```python
from build123d import *
from build123d.topology import SkipClean

# Parameters (mm, degrees)
SKETCH1_R           = 4.3
SKETCH1_R_2         = 3.5
BOSS_EXTRUDE1_DEPTH = 0.5
BOSS_EXTRUDE2_DEPTH = 2.5
SKETCH5_R           = 0.5
CUT_EXTRUDE2_DEPTH  = 3
CIRPATTERN1_COUNT   = 4


with BuildPart() as part:
    # Sketch1 → Boss-Extrude1 (new body)
    with BuildSketch(Plane.XY):
        Circle(SKETCH1_R)
        Circle(SKETCH1_R_2, mode=Mode.SUBTRACT)
    extrude(amount=BOSS_EXTRUDE1_DEPTH)

    # Sketch2 → Boss-Extrude2 (add)
    with SkipClean():  # the faces are left unmerged after this step: merging them gives an invalid solid
        with BuildSketch(Plane.XY.offset(0.5)):
            with BuildLine():
                Line((4.010922587, 1.55), (3.138072657, 1.55))
                ThreePointArc((3.138072657, 1.55), (2.474873734, 2.474873734), (1.55, 3.138072657))
                Line((1.55, 3.138072657), (1.55, 4.010922587))
                ThreePointArc((1.55, 4.010922587), (3.040559159, 3.040559159), (4.010922587, 1.55))
            make_face()
            with BuildLine():
                Line((-4.010922587, 1.55), (-3.138072657, 1.55))
                ThreePointArc((-3.138072657, 1.55), (-2.474873734, 2.474873734), (-1.55, 3.138072657))
                Line((-1.55, 3.138072657), (-1.55, 4.010922587))
                ThreePointArc((-1.55, 4.010922587), (-3.040559159, 3.040559159), (-4.010922587, 1.55))
            make_face()
            with BuildLine():
                Line((1.55, -4.010922587), (1.55, -3.138072657))
                ThreePointArc((1.55, -3.138072657), (2.474873734, -2.474873734), (3.138072657, -1.55))
                Line((3.138072657, -1.55), (4.010922587, -1.55))
                ThreePointArc((4.010922587, -1.55), (3.040559159, -3.040559159), (1.55, -4.010922587))
            make_face()
            with BuildLine():
                Line((-4.010922587, -1.55), (-3.138072657, -1.55))
                ThreePointArc((-3.138072657, -1.55), (-2.474873734, -2.474873734), (-1.55, -3.138072657))
                Line((-1.55, -3.138072657), (-1.55, -4.010922587))
                ThreePointArc((-1.55, -4.010922587), (-3.040559159, -3.040559159), (-4.010922587, -1.55))
            make_face()
        extrude(amount=BOSS_EXTRUDE2_DEPTH)

    # Sketch5 → Cut-Extrude2 (cut)
    with SkipClean():  # the faces are left unmerged after this step: merging them gives an invalid solid
        with BuildSketch(Plane(origin=(3.040559159, 3.040559159, 0), x_dir=(0, 0, -1), z_dir=(0.7071067811865499, 0.7071067811865452, 0))):
            with Locations(Location((-2.2, 0, 0), (0, 0, 90))):
                Circle(SKETCH5_R)
        cut_extrude2 = extrude(amount=-CUT_EXTRUDE2_DEPTH, mode=Mode.SUBTRACT)

    # CirPattern1: Cut-Extrude2 ×4 about axis
    with SkipClean():  # the faces are left unmerged after this step: merging them gives an invalid solid
        cirpattern1_axis = Axis((0, 0, 0.5), (0, 0, -1))
        for i in range(1, CIRPATTERN1_COUNT):
            add(cut_extrude2.rotate(cirpattern1_axis, i * 360 / CIRPATTERN1_COUNT), mode=Mode.SUBTRACT)


solid = part.part
```
The model under review builds one solid part; all positions refer to its coordinate system, in mm. A direction names the side the tool comes from. Coordinates: 2 decimals unless noted, no trailing zeros. Write each loop counter-clockwise with the first axis right and the second up, starting at its lowest first coordinate (ties: lowest second). Pieces come first, ordered by that corner, then holes.
1) Clearance check with flat-ended pins moving along their axes: pin 1 Ø1 at (y, z) = (4, 1.5) entering from -X; pin 2 Ø1.3 at (x, y) = (-4, -0.5) entering from +Z; pin 3 Ø1 at (y, z) = (1, 2) entering from +X; pin 4 Ø1 at (x, z) = (-3.5, 2) entering from +Y. State where each tip first meets the part, or that it passes through.
2) Machinability: for faces 1 (the face through (-2.8, -2.8, 3)), 2 (the face through (-1.55, -3.6, 1.7)), 3 (the face through (-4, 0, 0.5)), which of the approach directions +Z, -Z, +X, -X, +Y, -Y give a long, thin tool a straight path to every point of the face, cutting with its end or side? Answer none if there is none.
3) To check wall thickness, follow probe 1 along X at (y, z) = (-1.75, 0.45); probe 2 along X at (y, z) = (-1.5, 0.4); probe 3 along Z at (x, y) = (-4, -0.25). State the ranges of each line that lie inside material, in increasing order.
4) The part is to be moulded in two halves that separate along Y. For faces 4 (the face through (2.673, -2.826, 1.712)), 5 (the face through (1.55, 3.6, 1.7)), say which applies: pulls with the +Y half, pulls with the -Y half, needs draft (parallel to the pull), parting line crosses it, or undercut.
5) We need section A-A on z = 1.2. State the section outline as (x, y) points.
6) We need section B-B on x = 0. State the section outline as (y, z) points.
Answer list:
1. pin 1: stops at x = -2.5
1. pin 2: stops at z = 0.5
1. pin 3: passes through
1. pin 4: stops at y = 2.98
2. face 1: +Z, +X, -X, +Y, -Y
2. face 2: +Z, +Y, -Y
2. face 3: +Z, +X, -X
3. probe 1: x = -3.93 to -3.03, 3.03 to 3.93
3. probe 2: x = -4.03 to -3.16, 3.16 to 4.03
3. probe 3: z = 0 to 0.5
4. face 4: undercut
4. face 5: needs draft
5. outline: (-4.01, -1.55) arc R4.3 ccw to (-1.55, -4.01) - (-1.55, -3.14) arc R3.5 cw to (-3.14, -1.55) - close; (-4.01, 1.55) - (-3.14, 1.55) arc R3.5 cw to (-1.55, 3.14) - (-1.55, 4.01) arc R4.3 ccw to start; (1.55, -4.01) arc R4.3 ccw to (4.01, -1.55) - (3.14, -1.55) arc R3.5 cw to (1.55, -3.14) - close; (1.55, 3.14) arc R3.5 cw to (3.14, 1.55) - (4.01, 1.55) arc R4.3 ccw to (1.55, 4.01) - close
6. outline: (-4.3, 0) - (-3.5, 0) - (-3.5, 0.5) - (-4.3, 0.5) - close; (3.5, 0) - (4.3, 0) - (4.3, 0.5) - (3.5, 0.5) - close
